CAD build for the part. Positions are in the model's coordinates, mm. Face numbers are marked on the shaded views. Coordinates: 2 decimals unless noted, no trailing zeros. Write each loop counter-clockwise with the first axis right and the second up, starting at its lowest first coordinate (ties: lowest second). Pieces come first, ordered by that corner, then holes. Notation, with made-up numbers: (69.5, 29) -> (102.5, 29) arc R25 ccw to (102.5, 44) -> close; hole circle Ø1 at (5, 88). An arc over 180 degrees is marked (long way). Answer as CSV lines item,"result".
```python
from build123d import *

# Parameters (mm, degrees)
SKETCH1_W           = 90
SKETCH1_H           = 70
BOSS_EXTRUDE1_DEPTH = 1.6
SKETCH2_R           = 1.75
CUT_EXTRUDE1_DEPTH  = 58.031219521
CHAMFER1_SIZE       = 0.8


with BuildPart() as part:
    # Sketch1 → Boss-Extrude1 (new body)
    with BuildSketch(Plane(origin=(0, 0, 0), x_dir=(1, 0, 0), z_dir=(0, 1, 0))):
        Rectangle(SKETCH1_W, SKETCH1_H)
    extrude(amount=BOSS_EXTRUDE1_DEPTH)

    # Sketch2 → Cut-Extrude1 (cut, through all)
    with BuildSketch(Plane(origin=(0, 1.6, 0), x_dir=(1, 0, 0), z_dir=(0, 1, 0))):
        with Locations(Location((-40, -30, 0), (0, 0, 270))):
            Circle(SKETCH2_R)
        with Locations(Location((-40, 30, 0), (0, 0, 270))):
            Circle(SKETCH2_R)
        with Locations(Location((40, 30, 0), (0, 0, 270))):
            Circle(SKETCH2_R)
        with Locations(Location((40, -30, 0), (0, 0, 270))):
            Circle(SKETCH2_R)
    extrude(amount=-CUT_EXTRUDE1_DEPTH, mode=Mode.SUBTRACT)

    # Chamfer1
    chamfer1_edges = [part.edges().sort_by_distance(p)[0] for p in [
        (0, 1.6, 35),
        (0, 1.6, -35),
    ]]
    chamfer(chamfer1_edges, length=CHAMFER1_SIZE)


solid = part.part
```
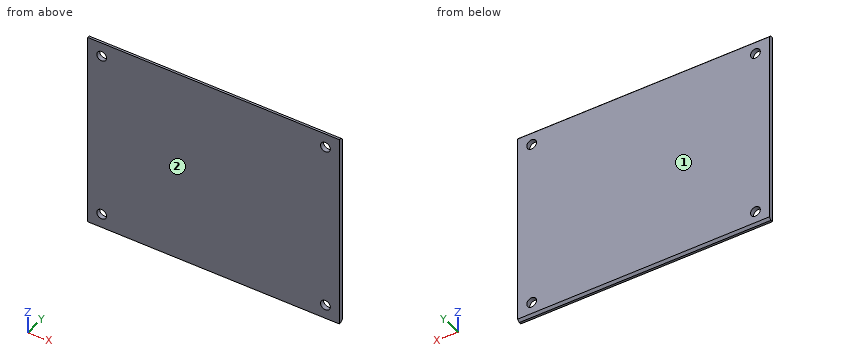
Item 1: Saw through at B-B on x = 40. Give the cut face in (y, z).
Answer below:
outline,"(0, -35) -> (0.8, -35) -> (1.6, -34.2) -> (1.6, -31.75) -> (0, -31.75) -> close; (0, -28.25) -> (1.6, -28.25) -> (1.6, 28.25) -> (0, 28.25) -> close; (0, 31.75) -> (1.6, 31.75) -> (1.6, 34.2) -> (0.8, 35) -> (0, 35) -> close"
Item 2: Wall check: line 1 (X direction, y = 0.9, z = -30); line 2 (X direction, y = 1, z = -31); line 3 (Z direction, x = 39, y = 0.75). Give the ranges that are in metal, low to high. Write a range as from..to.
Answer below:
line 1,"x = -45..-41.75, -38.25..38.25, 41.75..45"
line 2,"x = -45..-41.44, -38.56..38.56, 41.44..45"
line 3,"z = -35..-31.44, -28.56..28.56, 31.44..35"
Item 3: Saw through at C-C on y = 1.25. Give the cut face in (x, z).
Answer below:
outline,"(-45, -34.55) -> (45, -34.55) -> (45, 34.55) -> (-45, 34.55) -> close; hole circle Ø3.5 at (-40, -30); hole circle Ø3.5 at (-40, 30); hole circle Ø3.5 at (40, -30); hole circle Ø3.5 at (40, 30)"
Item 4: Saw through at A-A on z = -30. Give the cut face in (x, y).
Answer below:
outline,"(-45, 0) -> (-41.75, 0) -> (-41.75, 1.6) -> (-45, 1.6) -> close; (-38.25, 0) -> (38.25, 0) -> (38.25, 1.6) -> (-38.25, 1.6) -> close; (41.75, 0) -> (45, 0) -> (45, 1.6) -> (41.75, 1.6) -> close"
Item 5: Two-plate mould, pull along Y, no slides. Class the marked faces 1 and 2: pulls with the +Y half, pulls with the -Y half, needs draft (parallel to the pull), parting line crosses it, or undercut.
Answer below:
face 1,"pulls with the +Y half"
face 2,"pulls with the -Y half"
Item 6: Flat gauge pin, fed straight in: pin 1 (2 mm diameter, centred on x = 35, z = -27, fed in from -Y). Where does the tip first touch, or does it go through?
Answer below:
pin 1,"stops at y = 0"
